Source: CAD feature listing. Evaluate the final solid. Frame: model axes, mm. Coordinates: 2 decimals unless noted, no trailing zeros. Loops run counter-clockwise (first coordinate to the right, second up) from the corner with the lowest first, then second, coordinate; pieces in that order, holes last. Notation, with made-up numbers: M 12.25,73 L 71.25,73 A10 cw 71.25,78 Z; hole C -18.75,54.25 d5. An arc over 180 degrees is marked long. One line per question, with ' | ' between items. Start each with the question number.
1. Ray query, probe 1 along Y at (x, z) = (1.05, 0); probe 2 along Y at (x, z) = (1.1, 1); probe 3 along Z at (x, y) = (1.4, -69). Return the intervals inside material, ascending.
2. Section query A-A, the plane z = 0. Output: boundary loops of the cut face in (x, y).
3. Section query B-B, the plane x = 0.9. Output: boundary loops of the cut face in (y, z), and give its area (3 significant figures).
4. Pin query (flat end, axial travel): P1, Ø9.5, axis at y = 0, z = 0, coming from the -X side (1 decimal). Return the tip coordinate at first contact, or that it passes through.
5. Section query C-C, the plane y = -71.96. Output: boundary loops of the cut face in (x, z), and give its area (3 significant figures).
6. Section query D-D, the plane z = -26. Output: boundary loops of the cut face in (x, y).
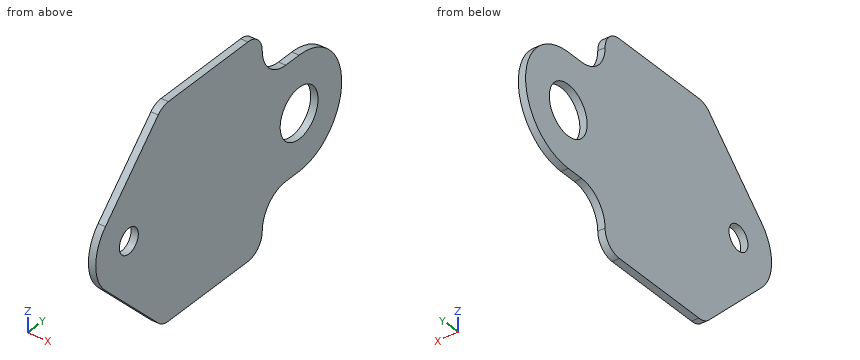
```python
from build123d import *

# Parameters (mm, degrees)
SKETCH1_R           = 8
SKETCH1_R_2         = 4
BOSS_EXTRUDE1_DEPTH = 2.3368


with BuildPart() as part:
    # Sketch1 → Boss-Extrude1 (new body)
    with BuildSketch(Plane(origin=(0, 0, 0), x_dir=(0, 0, -1), z_dir=(1, 0, 0))):
        with BuildLine():
            Line((-18, 0), (-18, -5.640538448))
            ThreePointArc((-18, -5.640538448), (-20.910261619, -12.666531518), (-27.936254688, -15.576793136))
            ThreePointArc((-27.936254688, -15.576793136), (-32.223970118, -17.352823019), (-34, -21.640538448))
            Line((-34, -21.640538448), (-34, -55.247304326))
            ThreePointArc((-34, -55.247304326), (-33.538424872, -57.567799195), (-32.223970118, -59.535019756))
            Line((-32.223970118, -59.535019756), (-9.899494937, -81.859494937))
            ThreePointArc((-9.899494937, -81.859494937), (0, -85.96), (9.899494937, -81.859494937))
            Line((9.899494937, -81.859494937), (32.223970118, -59.535019756))
            ThreePointArc((32.223970118, -59.535019756), (33.538424872, -57.567799195), (34, -55.247304326))
            Line((34, -55.247304326), (34, -21.640538448))
            ThreePointArc((34, -21.640538448), (32.223970118, -17.352823019), (27.936254688, -15.576793136))
            ThreePointArc((27.936254688, -15.576793136), (20.910261619, -12.666531518), (18, -5.640538448))
            Line((18, -5.640538448), (18, 0))
            ThreePointArc((18, 0), (0, 18), (-18, 0))
        make_face()
        Circle(SKETCH1_R, mode=Mode.SUBTRACT)
        with Locations((0, -71.96)):
            Circle(SKETCH1_R_2, mode=Mode.SUBTRACT)
    extrude(amount=BOSS_EXTRUDE1_DEPTH)


solid = part.part
```
Taken from the geometry:
1) probe 1: -85.96 to -75.96, -67.96 to -8, 8 to 18 | probe 2: -85.92 to -75.83, -68.09 to -7.94, 7.94 to 17.97 | probe 3: -22.76 to -2.69, 2.69 to 22.76
2) outline: M 0,-85.96 L 2.34,-85.96 L 2.34,-75.96 L 0,-75.96 Z; M 0,-67.96 L 2.34,-67.96 L 2.34,-8 L 0,-8 Z; M 0,8 L 2.34,8 L 2.34,18 L 0,18 Z
3) outline: M -81.86,-9.9 L -59.54,-32.22 A6.06 ccw -55.25,-34 L -21.64,-34 A6.06 ccw -15.58,-27.94 A9.94 cw -5.64,-18 L 0,-18 A18 ccw 0,18 L -5.64,18 A9.94 cw -15.58,27.94 A6.06 ccw -21.64,34 L -55.25,34 A6.06 ccw -59.54,32.22 L -81.86,9.9 A14 ccw Z; hole C -71.96,0 d8; hole C 0,0 d16 | area: 4,830 mm^2
4) P1: through
5) outline: M 0,-19.8 L 2.34,-19.8 L 2.34,-4 L 0,-4 Z; M 0,4 L 2.34,4 L 2.34,19.8 L 0,19.8 Z | area: 73.8 mm^2
6) outline: M 0,-65.76 L 2.34,-65.76 L 2.34,-15.39 L 0,-15.39 Z
